Source: three-view drawing plus pictorial views. Frame: mm from the lowest corner of the part. A direction names the side the tool comes from. Round coordinates to 2 decimals unless told otherwise and drop trailing zeros. Order: outer loops, then holes, each group sorted by start corner. A loop starts at its lowest first (then second) coordinate and runs counter-clockwise, first axis right, second up. Notation, with made-up numbers: (-0.5, 8.25) -> (4.5, 8.25) arc R17 ccw to (4.5, 32.25) -> close; hole circle Ø1 at (65, 42). An arc over 180 degrees is marked (long way). Answer as CSV lines item,"result".
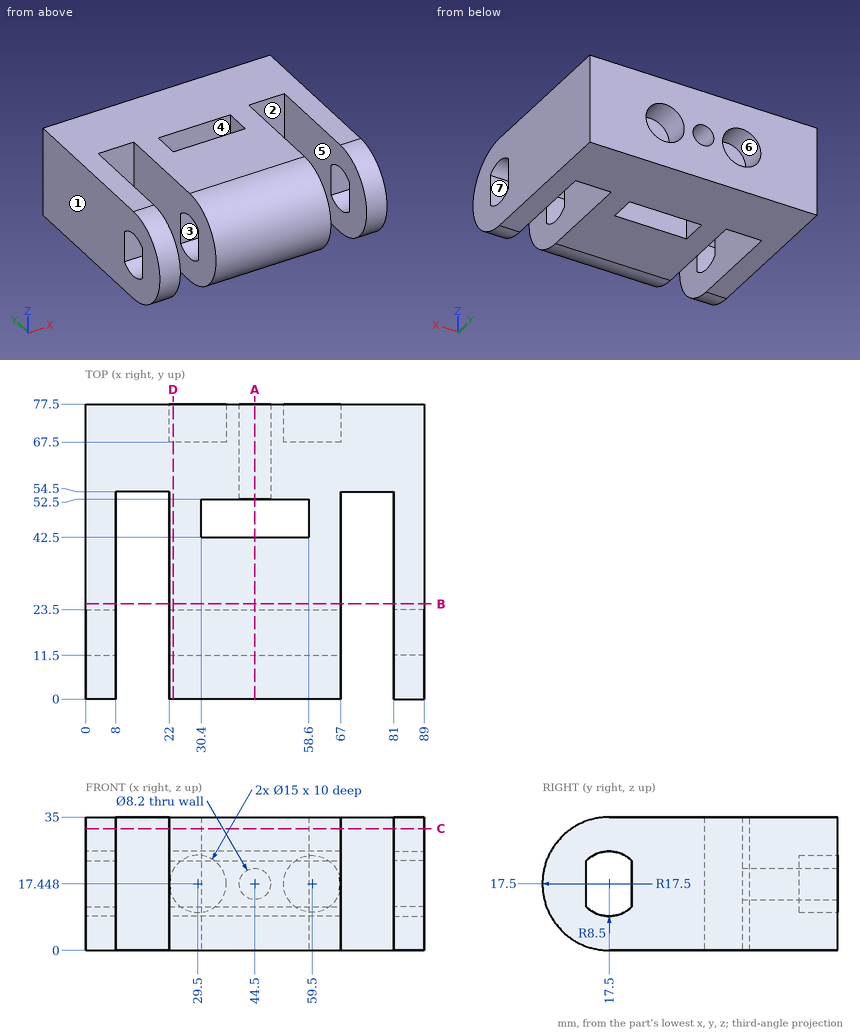
1. Mould query, pull axis X, two halves, no side actions, for the marked faces 1, 2, 3 and 4. Classes: released by +X, released by -X, zero draft, split by the parting line, or undercut.
Results below:
face 1,"released by -X"
face 2,"undercut"
face 3,"zero draft"
face 4,"undercut"
2. Pin query (flat end, axial travel): pin 1 (1 mm diameter, centred on x = 27, z = 25.5, fed in from -Y); pin 2 (9 mm diameter, centred on x = 59.5, z = 17.45, fed in from +Y). Return the tip coordinate at first contact, or that it passes through.
Results below:
pin 1,"y = 1.69"
pin 2,"y = 67.5"
3. Section query D-D on x = 23. Return loops of the section in (y, z), and give its area (3 significant figures).
Results below:
outline,"(17.5, 0) -> (77.5, 0) -> (77.5, 13.71) -> (67.5, 13.71) -> (67.5, 21.19) -> (77.5, 21.19) -> (77.5, 35) -> (17.5, 35) arc R17.5 ccw to start; hole (11.5, 11.48) arc R8.5 ccw to (23.5, 11.48) -> (23.5, 23.52) arc R8.5 ccw to (11.5, 23.52) -> close"
area,"2,320 mm2"
4. Section query A-A on x = 44.5. Return loops of the section in (y, z), and give its area (3 significant figures).
Results below:
outline,"(17.5, 0) -> (42.5, 0) -> (42.5, 35) -> (17.5, 35) arc R17.5 ccw to start; (52.5, 0) -> (77.5, 0) -> (77.5, 13.35) -> (52.5, 13.35) -> close; (52.5, 21.55) -> (77.5, 21.55) -> (77.5, 35) -> (52.5, 35) -> close; hole (11.5, 11.48) arc R8.5 ccw to (23.5, 11.48) -> (23.5, 23.52) arc R8.5 ccw to (11.5, 23.52) -> close"
area,"1,840 mm2"
5. Section query B-B on y = 25. Return loops of the section in (x, z).
Results below:
outline,"(0, 0) -> (8, 0) -> (8, 35) -> (0, 35) -> close; (22, 0) -> (67, 0) -> (67, 35) -> (22, 35) -> close; (81, 0) -> (89, 0) -> (89, 35) -> (81, 35) -> close"
6. Reachability of the marked faces 5, 6 and 7 from +Z, -Z, +X, -X, +Y, -Y: full face, straight path, thin tool, end or side. Return the list, or none.
Results below:
face 5,"+Z, -Z, -Y"
face 6,"+Y"
face 7,"+X, -X"
7. Section query C-C on z = 32. Return loops of the section in (x, y).
Results below:
outline,"(0, 7.7) -> (8, 7.7) -> (8, 54.5) -> (22, 54.5) -> (22, 7.7) -> (67, 7.7) -> (67, 54.5) -> (81, 54.5) -> (81, 7.7) -> (89, 7.7) -> (89, 77.5) -> (0, 77.5) -> close; hole (30.4, 42.5) -> (58.6, 42.5) -> (58.6, 52.5) -> (30.4, 52.5) -> close"
8. Line query: L1, parallel to X at y = 47.5, z = 2; L2, parallel to X at y = 39.5, z = 21.5; L3, parallel to Z at x = 29, y = 69 (1 decimal). Output: solid intervals per line, ascending. Write a range as [from, to].
Results below:
L1,"[0, 8], [22, 30.4], [58.6, 67], [81, 89]"
L2,"[0, 8], [22, 67], [81, 89]"
L3,"[0, 10], [24.9, 35]"
